from build123d import *

# Parameters (mm, degrees)
F0_W     = 28
F0_H     = 28
F1_DEPTH = 8
F2_R     = 7.5
F3_DEPTH = 15
F4_R     = 6
F5_DEPTH = 23.001


with BuildPart() as f1:
    # F0 (on Top) → F1 (new body)
    with BuildSketch(Plane.XY):
        Rectangle(F0_W, F0_H)
    extrude(amount=F1_DEPTH)

    # F2 (on face) → F3 (join)
    with BuildSketch(Plane(origin=(0, 0, 0), x_dir=(1, 0, 0), z_dir=(0, 0, -1))):
        Circle(F2_R)
    extrude(amount=F3_DEPTH)

    # F4 (on face) → F5 (cut, through all)
    with BuildSketch(Plane(origin=(0, 0, -15), x_dir=(1, 0, 0), z_dir=(0, 0, -1))):
        Circle(F4_R)
    extrude(amount=-F5_DEPTH, mode=Mode.SUBTRACT)


solid = f1.part
The listing builds one solid part. Answer for the finished solid, in the listing's coordinates (mm). Coordinates: 2 decimals unless noted, no trailing zeros. Order: outer loops, then holes, each group sorted by start corner. A loop starts at its lowest first (then second) coordinate and runs counter-clockwise, first axis right, second up.
Q1. A cutting plane is placed at C-C, the plane z = 4.5. Write down the section's boundary in (x, y).
Q2. A cutting plane is placed at A-A, the plane y = 0. Write down the section's boundary in (x, z).
Q3. For a pull along X with two mould halves and no side action, classify faces 1 (the face through (-6, -6, 0)), 2 (the face through (-6, 0, -4)), 3 (the face through (-7.493, -0.33, -7.395)) as pulls with the +X half, pulls with the -X half, needs draft (parallel to the pull), parting line crosses it, or undercut.
Q4. A cutting plane is placed at D-D, the plane x = 9.75. Write down the section's boundary in (y, z), and give its area (3 significant figures).
Q5. A cutting plane is placed at B-B, the plane x = 4.25. Write down the section's boundary in (y, z), and give its area (3 significant figures).
Q6. Consider line 1 (X direction, y = 0, z = -4.25); line 2 (Y direction, x = 0, z = 1.5). Determine where each line is inside the solid, lowest interval first.
Answers follow:
1. outline: (-14, -14) - (14, -14) - (14, 14) - (-14, 14) - close; hole circle Ø12 at (0, 0)
2. outline: (-14, 0) - (-7.5, 0) - (-7.5, -15) - (-6, -15) - (-6, 8) - (-14, 8) - close; (6, -15) - (7.5, -15) - (7.5, 0) - (14, 0) - (14, 8) - (6, 8) - close
3. face 1: needs draft
3. face 2: undercut
3. face 3: parting line crosses it
4. outline: (-14, 0) - (14, 0) - (14, 8) - (-14, 8) - close
4. area: 224 mm2
5. outline: (-14, 0) - (-6.18, 0) - (-6.18, -15) - (-4.24, -15) - (-4.24, 8) - (-14, 8) - close; (4.24, -15) - (6.18, -15) - (6.18, 0) - (14, 0) - (14, 8) - (4.24, 8) - close
5. area: 215 mm2
6. line 1: x = -7.5 to -6, 6 to 7.5
6. line 2: y = -14 to -6, 6 to 14
